from build123d import *

# Parameters (mm, degrees)
EXTRUDE_1_DEPTH     = 8
CUT_EXTRUDE_1_DEPTH = 8.6
EXTRUDE_2_DEPTH     = 8
EXTRUDE_3_DEPTH     = 10
SKETCH_7_R          = 5.75
CUT_EXTRUDE_2_DEPTH = 22
EXTRUDE_5_DEPTH     = 26
CUT_EXTRUDE_4_DEPTH = 21
CHAMFER_6_SIZE      = 5
CHAMFER_8_SIZE      = 10
SKETCH_13_W         = 210
SKETCH_13_H         = 10
CUT_EXTRUDE_5_DEPTH = 15
SKETCH_14_W         = 160
SKETCH_14_H         = 5
CUT_EXTRUDE_6_DEPTH = 10
SKETCH_16_R         = 2
CUT_EXTRUDE_7_DEPTH = 10
SKETCH_18_W         = 109.386418102
SKETCH_18_H         = 16
EXTRUDE_7_DEPTH     = 2
CHAMFER_10_SIZE     = 2


with BuildPart() as part:
    # 草图1 → 凸台-拉伸1 (new body)
    with BuildSketch(Plane.XY):
        Polygon((-60, 0), (60, 0), (115, 270), (-115, 270), align=None)
    extrude(amount=EXTRUDE_1_DEPTH)

    # 草图2 → 切除-拉伸1 (cut)
    with BuildSketch(Plane.XY.offset(8)):
        with BuildLine():
            Line((0.005000474, 0.310000947), (0, 0.3))
            Line((0, 0.3), (17.48870838, 0.3))
            Line((17.48870838, 0.3), (12.108893566, 26.71))
            Line((12.108893566, 26.71), (0, 26.71))
            ThreePointArc((0, 26.71), (-13.199999763, 13.507499763), (0.005000474, 0.310000947))
        make_face()
    extrude(amount=-CUT_EXTRUDE_1_DEPTH, mode=Mode.SUBTRACT)

    # 草图5 → 凸台-拉伸2 (add)
    with BuildSketch(Plane(origin=(0, 0, 0), x_dir=(-1, 0, 0), z_dir=(0, 0, -1))):
        Polygon((60, 0), (115, 270), (-115, 270), (-60, 0), align=None)
    extrude(amount=EXTRUDE_2_DEPTH)

    # 草图6 → 凸台-拉伸3 (add)
    with BuildSketch(Plane.XY.offset(8)):
        Polygon((-115, 270), (-60, 0), (60, 0), (115, 270), align=None)
    extrude(amount=EXTRUDE_3_DEPTH)

    # 草图7 → 切除-拉伸2 (cut)
    with BuildSketch(Plane.XY.offset(18)):
        with Locations((0, 13.51)):
            Circle(SKETCH_7_R)
    extrude(amount=-CUT_EXTRUDE_2_DEPTH, mode=Mode.SUBTRACT)

    # 草图9 → 凸台-拉伸5 (add)
    with BuildSketch(Plane.XY.offset(18)):
        Polygon((-57.962962963, -10), (-60, 0), (60, 0), (57.962962963, -10), align=None)
    extrude(amount=-EXTRUDE_5_DEPTH)

    # 草图12 → 切除-拉伸4 (cut)
    with BuildSketch(Plane.XY.offset(-8)):
        Polygon((54.693209051, 0), (-54.693209051, 0), (-52.656172014, -10), (52.656172014, -10), align=None)
    extrude(amount=CUT_EXTRUDE_4_DEPTH, mode=Mode.SUBTRACT)

    # 倒角6
    chamfer_6_edges = [part.edges().sort_by_distance(p)[0] for p in [
        (0, 0, -8),
    ]]
    chamfer(chamfer_6_edges, length=CHAMFER_6_SIZE)

    # 倒角8
    chamfer_8_edges = [part.edges().sort_by_distance(p)[0] for p in [
        (55.309567488, -10, -8),
        (-55.309567488, -10, -8),
    ]]
    chamfer(chamfer_8_edges, length=CHAMFER_8_SIZE)

    # 草图13 → 切除-拉伸5 (cut)
    with BuildSketch(Plane(origin=(0, 270, 0), x_dir=(1, 0, 0), z_dir=(0, 1, 0))):
        with Locations((0, -5)):
            Rectangle(SKETCH_13_W, SKETCH_13_H)
    extrude(amount=-CUT_EXTRUDE_5_DEPTH, mode=Mode.SUBTRACT)

    # 草图14 → 切除-拉伸6 (cut)
    with BuildSketch(Plane.XY.offset(18)):
        with Locations((0, 173.51)):
            Rectangle(SKETCH_14_W, SKETCH_14_H)
    extrude(amount=-CUT_EXTRUDE_6_DEPTH, mode=Mode.SUBTRACT)

    # 草图16 → 切除-拉伸7 (cut)
    with BuildSketch(Plane.XY.offset(18)):
        with BuildLine():
            ThreePointArc((-88.677124344, 235), (-90, 238.5), (-91.322875656, 235))
            Line((-91.322875656, 235), (-88.677124344, 235))
        make_face()
        with BuildLine():
            ThreePointArc((91.322875656, 235), (90, 238.5), (88.677124344, 235))
            Line((88.677124344, 235), (91.322875656, 235))
        make_face()
        with BuildLine():
            ThreePointArc((65.822875656, 235), (64.5, 238.5), (63.177124344, 235))
            Line((63.177124344, 235), (65.822875656, 235))
        make_face()
        with BuildLine():
            ThreePointArc((-63.177124344, 235), (-64.5, 238.5), (-65.822875656, 235))
            Line((-65.822875656, 235), (-63.177124344, 235))
        make_face()
        with Locations((-77.25, 255.6425573)):
            Circle(SKETCH_16_R)
        with Locations((77.25, 255.6425573)):
            Circle(SKETCH_16_R)
        with Locations((-55, 154.1525573)):
            Circle(SKETCH_16_R)
        with Locations((-67.75, 135.01)):
            Circle(SKETCH_16_R)
        with Locations((-42.25, 135.01)):
            Circle(SKETCH_16_R)
        with Locations((42.25, 135.01)):
            Circle(SKETCH_16_R)
        with Locations((67.75, 135.01)):
            Circle(SKETCH_16_R)
        with Locations((55, 154.1525573)):
            Circle(SKETCH_16_R)
    extrude(amount=-CUT_EXTRUDE_7_DEPTH, mode=Mode.SUBTRACT)

    # 草图18 → 凸台-拉伸7 (add)
    with BuildSketch(Plane.XZ):
        with Locations((0, 5)):
            Rectangle(SKETCH_18_W, SKETCH_18_H)
    extrude(amount=EXTRUDE_7_DEPTH)

    # 倒角10
    chamfer_10_edges = [part.edges().sort_by_distance(p)[0] for p in [
        (0, -2, -3),
    ]]
    chamfer(chamfer_10_edges, length=CHAMFER_10_SIZE - 0.0001)  # a hair under: the kernel refuses the full size


solid = part.part
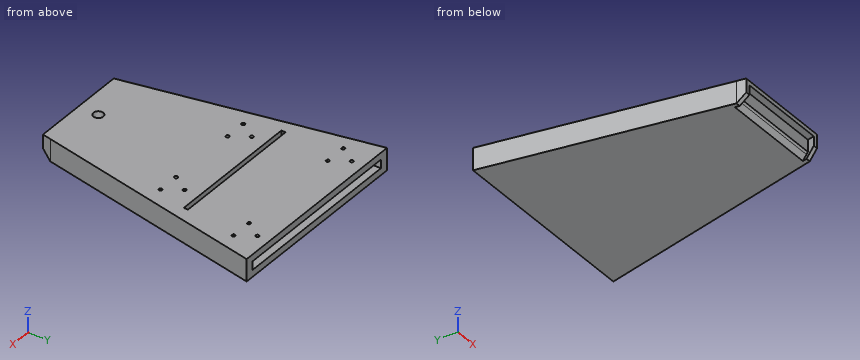
Could you check a few things on this model? Use its own coordinates, in mm. Round coordinates to 2 decimals unless told otherwise and drop trailing zeros. Write each loop counter-clockwise with the first axis right and the second up, starting at its lowest first coordinate (ties: lowest second). Pieces come first, ordered by that corner, then holes. Notation, with made-up numbers: (42, -4) -> (63, -4) arc R14 ccw to (63, 4) -> close; hole circle Ø11 at (88.25, -13). An arc over 180 degrees is marked (long way). Use a Markdown table: item, result.
1. For pin 1 Ø1 at (y, z) = (205, 10.5) entering from +X; pin 2 Ø7 at (x, z) = (15, 6) entering from -Y; pin 3 Ø9 at (x, y) = (12, -5.5) entering from -Z, each with a flat end and sliding along its axis, tell me the tip position at first contact or that it passes through.
Answer key:
| item | result |
|---|---|
| pin 1 | stops at x = 101.86 |
| pin 2 | stops at y = -2 |
| pin 3 | stops at z = -2 |
2. If we section it at B-B (y = 13.51): List the corners of the cut face in (x, z) for me, then the cut area to 3 significant figures.
Answer key:
| item | result |
|---|---|
| outline | (-62.75, -8) -> (62.75, -8) -> (62.75, 18) -> (5.75, 18) -> (5.75, 8) -> (14.8, 8) -> (14.8, 0) -> (5.75, 0) -> (5.75, -4) -> (-5.75, -4) -> (-5.75, 0) -> (-13.2, 0) -> (-13.2, 8) -> (-5.75, 8) -> (-5.75, 18) -> (-62.75, 18) -> close |
| area | 2,880 mm^2 |
3. If we section it at D-D (y = 110): List the corners of the cut face in (x, z) for me.
Answer key:
| item | result |
|---|---|
| outline | (-82.41, -8) -> (82.41, -8) -> (82.41, 18) -> (-82.41, 18) -> close |
4. If we section it at C-C (x = 96): List the corners of the cut face in (y, z) for me.
Answer key:
| item | result |
|---|---|
| outline | (176.73, -8) -> (270, -8) -> (270, 0) -> (255, 0) -> (255, 10) -> (270, 10) -> (270, 18) -> (176.73, 18) -> close |
5. Please list where these lines run through material, in increasing order: probe 1 along X at (y, z) = (236.5, 15.25); probe 2 along X at (y, z) = (135.01, 12.25); probe 3 along Z at (x, y) = (2.5, 25.5).
Answer key:
| item | result |
|---|---|
| probe 1 | x = -108.18 to -92, -88 to -66.5, -62.5 to 62.5, 66.5 to 88, 92 to 108.18 |
| probe 2 | x = -87.5 to -69.75, -65.75 to -44.25, -40.25 to 40.25, 44.25 to 65.75, 69.75 to 87.5 |
| probe 3 | z = -8 to 0, 8 to 18 |
